from build123d import *

# Parameters (mm, degrees)
SKETCH1_W               = 16
SKETCH1_H               = 12
BOSS_EXTRUDE1_DEPTH     = 7
SKETCH2_W               = 13
SKETCH2_H               = 10
CUT_EXTRUDE1_DEPTH      = 18.204650534
SKETCH6_W               = 10
SKETCH6_H               = 10
BOSS_EXTRUDE2_DEPTH     = 3
FILLET1_R               = 0.5
CUT_EXTRUDE2_DEPTH      = 22.307275753
CUT_EXTRUDE2_DEPTH_BACK = 10
SKETCH9_R               = 2.05


with BuildPart() as part:
    # Sketch1 → Boss-Extrude1 (new, symmetric)
    with BuildSketch(Plane.XY):
        Rectangle(SKETCH1_W, SKETCH1_H)
    extrude(amount=BOSS_EXTRUDE1_DEPTH, both=True)

    # Sketch2 → Cut-Extrude1 (cut, through all)
    with BuildSketch(Plane.XY.offset(7)):
        with Locations((0, -1)):
            Rectangle(SKETCH2_W, SKETCH2_H)
    extrude(amount=-CUT_EXTRUDE1_DEPTH, mode=Mode.SUBTRACT)

    # Sketch6 → Boss-Extrude2 (add)
    with BuildSketch(Plane.XZ.offset(6)):
        with Locations((-13, 0)):
            Rectangle(SKETCH6_W, SKETCH6_H)
        with Locations((13, 0)):
            Rectangle(SKETCH6_W, SKETCH6_H)
    extrude(amount=-BOSS_EXTRUDE2_DEPTH)

    # Fillet1
    fillet1_edges = [part.edges().sort_by_distance(p)[0] for p in [
        (-8, -4.5, 5),
        (-8, -4.5, -5),
        (-8, -3, 0),
        (8, -4.5, -5),
        (8, -4.5, 5),
        (8, -3, 0),
        (-8, 6, 0),
        (8, 6, 0),
    ]]
    fillet(fillet1_edges, radius=FILLET1_R)

    # Sketch9 → Cut-Extrude2 (cut, two sides: drawn at the far end of the back side and taken through both)
    with BuildSketch(Plane(origin=(0, -3, 0), x_dir=(1, 0, 0), z_dir=(0, 1, 0)).offset(-CUT_EXTRUDE2_DEPTH_BACK)):
        with Locations(Location((-14.25, 0, 0), (0, 0, 90))):
            Circle(SKETCH9_R)
        with Locations(Location((14.25, 0, 0), (0, 0, 90))):
            Circle(SKETCH9_R)
    extrude(amount=CUT_EXTRUDE2_DEPTH + CUT_EXTRUDE2_DEPTH_BACK, mode=Mode.SUBTRACT)


solid = part.part
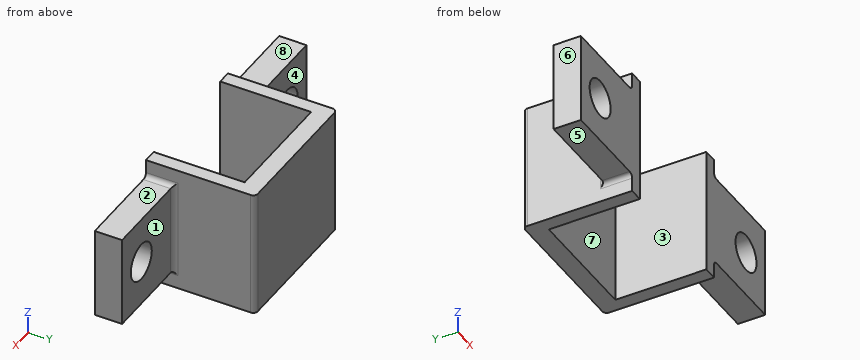
Check sheet for the modelled part. Datum: model origin and axes. Units: mm. Face numbers are marked on the shaded views. A direction names the side the tool comes from. Round coordinates to 2 decimals unless told otherwise and drop trailing zeros. Order: outer loops, then holes, each group sorted by start corner. A loop starts at its lowest first (then second) coordinate and runs counter-clockwise, first axis right, second up. Notation, with made-up numbers: M 46.5,-3 L 98.5,-3 A32 ccw 98.5,36 Z; hole C -22,5.25 d8. An arc over 180 degrees is marked long. One line per item, written item: value. Start each with the question number.
1. Section check A-A on x = 14.25. Enter the section's corners in (y, z).
2. Gauge pin test, flat ends, axial feed: P1, Ø5, axis at x = -13.5, z = 0, coming from the +Y side; P2, Ø0.9, axis at x = -13.5, y = -4.5, coming from the +Z side; P3, Ø3.5, axis at x = -15.5, y = -5, coming from the -Z side; P4, Ø3.5, axis at x = -14.25, z = 0, coming from the -Y side. Record the tip position at first contact, or that the pin passes through.
3. Access from +Z, -Z, +X, -X, +Y, -Y to the whole of each face (thin tool, end or side, straight path). Record for the marked faces 1, 2, 3, 4 and 5.
4. Release check for a two-part mould opening along X. For the marked faces 6, 7 and 8 record: released by +X, released by -X, zero draft, split by the parting line, or undercut.
5. Section check C-C on z = 0. Enter the section's corners in (x, y), and give its area (3 significant figures).
6. Section check B-B on y = 2.25. Enter the section's corners in (x, z), and give its area (3 significant figures).
7. Section check D-D on z = 4.5. Enter the section's corners in (x, y), and give its area (3 significant figures).
8. Scan lines: line 1 along X through (y, z) = (-4.7, 0); line 2 along X through (y, z) = (-0.75, 3.5); line 3 along X through (y, z) = (-4, 1.5). Record each from-to range of solid material in increasing order.
Results found:
1. outline: M -6,-5 L -3,-5 L -3,-2.05 L -6,-2.05 Z; M -6,2.05 L -3,2.05 L -3,5 L -6,5 Z
2. P1: y = -3
2. P2: z = 5
2. P3: z = -5
2. P4: through
3. face 1: +Z, -Z, +X, +Y
3. face 2: +Z, +X, +Y, -Y
3. face 3: +Z, -Z, -Y
3. face 4: +Z, -Z, -X, +Y
3. face 5: -Z, -X, +Y, -Y
4. face 6: released by -X
4. face 7: undercut
4. face 8: zero draft
5. outline: M -18,-6 L -16.3,-6 L -16.3,-3 L -18,-3 Z; M -12.2,-6 L -6.5,-6 L -6.5,4 L 6.5,4 L 6.5,-6 L 12.2,-6 L 12.2,-3 L 8.5,-3 A0.5 cw 8,-2.5 L 8,5.5 A0.5 ccw 7.5,6 L -7.5,6 A0.5 ccw -8,5.5 L -8,-2.5 A0.5 cw -8.5,-3 L -12.2,-3 Z; M 16.3,-6 L 18,-6 L 18,-3 L 16.3,-3 Z
5. area: 97.4 mm^2
6. outline: M -8,-7 L -6.5,-7 L -6.5,7 L -8,7 Z; M 6.5,-7 L 8,-7 L 8,7 L 6.5,7 Z
6. area: 42.0 mm^2
7. outline: M -18,-6 L -6.5,-6 L -6.5,4 L 6.5,4 L 6.5,-6 L 18,-6 L 18,-3 L 8.5,-3 A0.5 cw 8,-2.5 L 8,5.5 A0.5 ccw 7.5,6 L -7.5,6 A0.5 ccw -8,5.5 L -8,-2.5 A0.5 cw -8.5,-3 L -18,-3 Z
7. area: 122 mm^2
8. line 1: -18 to -16.3, -12.2 to -6.5, 6.5 to 12.2, 16.3 to 18
8. line 2: -8 to -6.5, 6.5 to 8
8. line 3: -18 to -15.65, -12.85 to -6.5, 6.5 to 12.85, 15.65 to 18
